Input: part model. Units: mm. Frame: model coordinates. A direction names the side the tool comes from. Round coordinates to 2 decimals unless told otherwise and drop trailing zeros. Loops run counter-clockwise (first coordinate to the right, second up) from the corner with the lowest first, then second, coordinate; pieces in that order, holes last. Notation, with made-up numbers: M 17.5,25.5 L 23.5,25.5 A11 cw 23.5,39.5 Z; hole C 89,-21 d6. An arc over 180 degrees is marked long. Put each result on its own line as item: value. Start each with the question number.
1) Section A-A on y = -5. Output: boundary loops of the cut face in (x, z).
2) Draft query along Z for faces 1 (the face through (1.97, -5.26, -6.88)), 2 (the face through (1.972, 2.786, 8.194)), 3 (the face through (0, -4, 0)), 4 (the face through (1.97, -2.74, -8.19)). Return one class per face: +Z half, -Z half, draft (parallel to the pull), parting line (faces both ways), or undercut.
3) Line query: probe 1 along Y at (x, z) = (-0.25, 0); probe 2 along Z at (x, y) = (-0.4, 0); probe 3 along Z at (x, y) = (2.3, 6.75). Output: solid intervals per line, ascending.
4) Pin query (flat end, axial travel): pin 1 (4.5 mm diameter, centred on y = 0, z = 0, fed in from +X); pin 2 (0.5 mm diameter, centred on x = 2.5, y = 2.5, fed in from +Z); pin 3 (1 mm diameter, centred on y = 6.5, z = 6, fed in from -X); pin 4 (3 mm diameter, centred on x = 1, y = 7.5, fed in from -Z). Return the tip coordinate at first contact, or that it passes through.
5) Reachability of faces 5 (the face through (1.97, 7.18, 4.84)), 6 (the face through (1.972, 8.333, -2.339)), 7 (the face through (1.97, -3.66, -7.85)), 8 (the face through (1.97, 4.48, 7.4)) from +Z, -Z, +X, -X, +Y, -Y: full face, straight path, thin tool, end or side. Return the list, or none.
from build123d import *
from build123d.topology import SkipClean

# Parameters (mm, degrees)
BASPROSKE_W             = 4
BASPROSKE_H             = 9.3
TOOTHCUT_DEPTH          = 14.746999673
TEETHCUTS_COUNT         = 29
TEETHCUTS_ANGLE         = 347.586206897
BORSKE_R                = 2.5
BORE_DEPTH              = 50.0000508
EXTRUDE1_DEPTH          = 4.5
EXTRUDE1_DEPTH_BACK     = 0.5
SKETCH1_R               = 3.25
SKETCH1_R_2             = 2.5
CUT_EXTRUDE1_DEPTH      = 20
CUT_EXTRUDE1_DEPTH_BACK = 14.896807231
SKETCH2_W               = 1.5
SKETCH2_H               = 2.8


with BuildPart() as part:
    # BasProSke → Base-Revolve (revolve)
    with BuildSketch(Plane(origin=(0, 0, 0), x_dir=(1, 0, 0), z_dir=(0, 1, 0)), mode=Mode.PRIVATE) as base_revolve_sk:
        with Locations((2, 4.65)):
            Rectangle(BASPROSKE_W, BASPROSKE_H)
    revolve(base_revolve_sk.sketch.rotate(Axis((-10, 0, 0), (1, 0, 0)), 180), axis=Axis((-10, 0, 0), (1, 0, 0)))

    # TooCutSke → ToothCut (cut, through all)
    with BuildSketch(Plane(origin=(0, 0, 0), x_dir=(0, 0, -1), z_dir=(1, 0, 0))):
        with BuildLine():
            ThreePointArc((0.281517973, 7.944013383), (0, 7.949), (-0.281517973, 7.944013383))
            ThreePointArc((-0.281517973, 7.944013383), (-0.494228582, 8.645390123), (-0.84911719, 9.28666168))
            ThreePointArc((-0.84911719, 9.28666168), (0, 9.3254), (0.84911719, 9.28666168))
            ThreePointArc((0.84911719, 9.28666168), (0.494228582, 8.645390123), (0.281517973, 7.944013383))
        make_face()
    toothcut = extrude(amount=TOOTHCUT_DEPTH, mode=Mode.SUBTRACT)

    # TeethCuts: ToothCut ×29 about axis
    teethcuts_axis = Axis((-10, 0, 0), (1, 0, 0))
    for i in range(1, TEETHCUTS_COUNT):
        add(toothcut.rotate(teethcuts_axis, i * TEETHCUTS_ANGLE / (TEETHCUTS_COUNT - 1)), mode=Mode.SUBTRACT)

    # BorSke → Bore (cut, symmetric)
    with BuildSketch(Plane(origin=(0, 0, 0), x_dir=(0, 0, -1), z_dir=(1, 0, 0))):
        with Locations(Location((0, 0, 0), (0, 0, 180))):
            Circle(BORSKE_R)
    extrude(amount=BORE_DEPTH, both=True, mode=Mode.SUBTRACT)

    # Sketch1 → Extrude1 (add, two sides: drawn at the far end of the back side and taken through both)
    with SkipClean():  # the faces are left unmerged after this step: merging them gives an invalid solid
        with BuildSketch(Plane(origin=(0, 0, 0), x_dir=(0, 0, -1), z_dir=(1, 0, 0)).offset(-EXTRUDE1_DEPTH_BACK)):
            Circle(SKETCH1_R)
            Circle(SKETCH1_R_2, mode=Mode.SUBTRACT)
        extrude(amount=EXTRUDE1_DEPTH + EXTRUDE1_DEPTH_BACK)
    add(part.part.scale(1), mode=Mode.REPLACE)  # the faces are merged on a copy

    # Sketch2 → Cut-Extrude1 (cut, two sides: drawn at the far end of the back side and taken through both)
    with SkipClean():  # the faces are left unmerged after this step: merging them gives an invalid solid
        with BuildSketch(Plane(origin=(0, 0, 0), x_dir=(0, 0, -1), z_dir=(1, 0, 0)).offset(-CUT_EXTRUDE1_DEPTH_BACK)):
            with Locations((0, 1.4)):
                Rectangle(SKETCH2_W, SKETCH2_H)
        extrude(amount=CUT_EXTRUDE1_DEPTH + CUT_EXTRUDE1_DEPTH_BACK, mode=Mode.SUBTRACT)


solid = part.part
Geometry results:
1. outline: M 0,-6.69 L 4,-6.69 L 4,6.69 L 0,6.69 Z
2. face 1: -Z half
2. face 2: +Z half
2. face 3: draft
2. face 4: undercut
3. probe 1: y = -3.25 to -2.5, 2.8 to 3.25
3. probe 2: z = -3.25 to -2.5, 2.5 to 3.25
3. probe 3: z = -6.4 to -5.96, -4.7 to 4.7, 5.96 to 6.4
4. pin 1: passes through
4. pin 2: stops at z = 8.15
4. pin 3: stops at x = 0
4. pin 4: stops at z = -6.52
5. face 5: +X, -X
5. face 6: +X, -X, +Y
5. face 7: -Z, +X, -X
5. face 8: +Z, +X, -X
